Part model, mm, in its own coordinate system. A direction names the side the tool comes from. Coordinates: 2 decimals unless noted, no trailing zeros. Order: outer loops, then holes, each group sorted by start corner. A loop starts at its lowest first (then second) coordinate and runs counter-clockwise, first axis right, second up.
from build123d import *

# Parameters (mm, degrees)
SKETCH_4_W          = 233.6
SKETCH_4_H          = 150
EXTRUDE_2_DEPTH     = 2.2
SKETCH_6_W          = 2
SKETCH_6_H          = 10
EXTRUDE_3_DEPTH     = 1.8
SKETCH_7_W          = 233.6
SKETCH_7_H          = 6
EXTRUDE_4_DEPTH     = 5
SKETCH_8_W          = 114.8
SKETCH_8_H          = 2.2
SKETCH_8_W_2        = 116.8
SKETCH_8_W_3        = 231.6
CUT_EXTRUDE_1_DEPTH = 3


with BuildPart() as part:
    # 草图4 → 凸台-拉伸2 (new body)
    with BuildSketch(Plane(origin=(0, 0, 0), x_dir=(0, 0, -1), z_dir=(1, 0, 0))):
        Rectangle(SKETCH_4_W, SKETCH_4_H)
    extrude(amount=EXTRUDE_2_DEPTH)

    # 草图6 → 凸台-拉伸3 (add)
    with BuildSketch(Plane.XZ.offset(75)):
        with Locations((1.1, 20)):
            Rectangle(SKETCH_6_W, SKETCH_6_H)
        with Locations((1.1, 0)):
            Rectangle(SKETCH_6_W, SKETCH_6_H)
        with Locations((1.1, 40)):
            Rectangle(SKETCH_6_W, SKETCH_6_H)
        with Locations((1.1, 60)):
            Rectangle(SKETCH_6_W, SKETCH_6_H)
        with Locations((1.1, 80)):
            Rectangle(SKETCH_6_W, SKETCH_6_H)
        with Locations((1.1, 100)):
            Rectangle(SKETCH_6_W, SKETCH_6_H)
        with Locations((1.1, -20)):
            Rectangle(SKETCH_6_W, SKETCH_6_H)
        with Locations((1.1, -40)):
            Rectangle(SKETCH_6_W, SKETCH_6_H)
        with Locations((1.1, -60)):
            Rectangle(SKETCH_6_W, SKETCH_6_H)
        with Locations((1.1, -80)):
            Rectangle(SKETCH_6_W, SKETCH_6_H)
        with Locations((1.1, -100)):
            Rectangle(SKETCH_6_W, SKETCH_6_H)
    extrude(amount=EXTRUDE_3_DEPTH)

    # 草图7 → 凸台-拉伸4 (add)
    with BuildSketch(Plane(origin=(2.2, 0, 0), x_dir=(0, 0, -1), z_dir=(1, 0, 0))):
        with Locations((0, 28)):
            Rectangle(SKETCH_7_W, SKETCH_7_H)
        with Locations((0, 72)):
            Rectangle(SKETCH_7_W, SKETCH_7_H)
    extrude(amount=EXTRUDE_4_DEPTH)

    # 草图8 → 切除-拉伸1 (cut)
    with BuildSketch(Plane(origin=(7.2, 0, 0), x_dir=(0, 0, -1), z_dir=(1, 0, 0))):
        with Locations((-57.4, 28)):
            Rectangle(SKETCH_8_W, SKETCH_8_H)
        with Locations((58.4, 28)):
            Rectangle(SKETCH_8_W_2, SKETCH_8_H)
        with Locations((1, 72)):
            Rectangle(SKETCH_8_W_3, SKETCH_8_H)
    extrude(amount=-CUT_EXTRUDE_1_DEPTH, mode=Mode.SUBTRACT)


solid = part.part
Q1. Cut at C-C on z = -31.5. Write the cut outline in (x, y), and give its area (3 significant figures).
Results list:
outline: (0, -75) - (2.2, -75) - (2.2, 25) - (7.2, 25) - (7.2, 26.9) - (4.2, 26.9) - (4.2, 29.1) - (7.2, 29.1) - (7.2, 31) - (2.2, 31) - (2.2, 69) - (7.2, 69) - (7.2, 70.9) - (4.2, 70.9) - (4.2, 73.1) - (7.2, 73.1) - (7.2, 75) - (0, 75) - close
area: 377 mm2
Q2. Pin check, flat tips, straight feed: pin 1 Ø0.5 at (y, z) = (-76, -38) entering from -X; pin 2 Ø0.5 at (y, z) = (-75.5, 19.5) entering from +X; pin 3 Ø6 at (y, z) = (54.5, 24.5) entering from +X. Stop position of each tip, or through.
Results list:
pin 1: stops at x = 0.1
pin 2: stops at x = 2.1
pin 3: stops at x = 2.2
Q3. Cut at B-B on z = 22. Write the cut outline in (x, y), and give its area (3 significant figures).
Results list:
outline: (0, -75) - (0.1, -75) - (0.1, -76.8) - (2.1, -76.8) - (2.1, -75) - (2.2, -75) - (2.2, 25) - (7.2, 25) - (7.2, 26.9) - (4.2, 26.9) - (4.2, 29.1) - (7.2, 29.1) - (7.2, 31) - (2.2, 31) - (2.2, 69) - (7.2, 69) - (7.2, 70.9) - (4.2, 70.9) - (4.2, 73.1) - (7.2, 73.1) - (7.2, 75) - (0, 75) - close
area: 380 mm2
Q4. Cut at A-A on x = 5.5. Write the cut outline in (y, z), and give its area (3 significant figures).
Results list:
outline: (25, -116.8) - (26.9, -116.8) - (26.9, 114.8) - (29.1, 114.8) - (29.1, -116.8) - (31, -116.8) - (31, 116.8) - (25, 116.8) - close; (69, -116.8) - (70.9, -116.8) - (70.9, 114.8) - (73.1, 114.8) - (73.1, -116.8) - (75, -116.8) - (75, 116.8) - (69, 116.8) - close
area: 1,780 mm2
Q5. Which spindle directions (+Z, -Z, +X, -X, +Y, -Y) get a long thin tool onto all of the face, cutting with end or side? Do faces 4 (the face through (2.2, -24, 2)), 5 (the face through (2, 5, 116.8)), 6 (the face through (5, 31, 2)). Say none if no direction does.
Results list:
face 4: +Z, -Z, +X, -Y
face 5: +Z, +X, -X, +Y, -Y
face 6: +Z, -Z, +X
Q6. Wall check: line 1 along Y through (x, z) = (5.25, 71); line 2 along Y through (x, z) = (3.75, 76); line 3 along X through (y, z) = (5.5, 82.5). Give the ranges that are in metal, low to high.
Results list:
line 1: y = 25 to 26.9, 29.1 to 31, 69 to 70.9, 73.1 to 75
line 2: y = 25 to 31, 69 to 75
line 3: x = 0 to 2.2
Q7. Mould opens along Y. For faces 1 (the face through (2.2, 50, 2)), 2 (the face through (5, 25, 2)), 3 (the face through (4, 75, 2)) say: pulls with the +Y half, pulls with the -Y half, needs draft (parallel to the pull), parting line crosses it, or undercut.
Results list:
face 1: undercut
face 2: pulls with the -Y half
face 3: pulls with the +Y half
Q8. Cut at D-D on y = 54. Write the cut outline in (x, z).
Results list:
outline: (0, -116.8) - (2.2, -116.8) - (2.2, 116.8) - (0, 116.8) - close
